```python
from build123d import *

# Parameters (mm, degrees)
F0_W     = 270
F0_H     = 270
F1_DEPTH = 240
F2_R     = 20
F3_T     = -2.5


with BuildPart() as f1:
    # F0 (on Top) → F1 (new body)
    with BuildSketch(Plane.XY):
        with Locations((137.330786, 0)):
            Rectangle(F0_W, F0_H)
    extrude(amount=-F1_DEPTH)

    # F2
    f2_edges = [f1.edges().sort_by_distance(p)[0] for p in [
        (137.330786, -135, -240),
        (272.330786, 0, -240),
        (137.330786, 135, -240),
        (2.330786, 0, -240),
        (2.330786, -135, -120),
        (272.330786, -135, -120),
        (272.330786, 135, -120),
        (2.330786, 135, -120),
    ]]
    fillet(f2_edges, radius=F2_R)

    # F3
    f3_openings = [f1.faces().sort_by_distance(p)[0] for p in [
        (137.330786, 0, 0),
    ]]
    offset(amount=F3_T, openings=f3_openings)


solid = f1.part
```
The listing builds one solid part. Answer for the finished solid, in the listing's coordinates (mm). A direction names the side the tool comes from. Coordinates: 2 decimals unless noted, no trailing zeros. Loops run counter-clockwise (first coordinate to the right, second up) from the corner with the lowest first, then second, coordinate; pieces in that order, holes last. Notation, with made-up numbers: (8.25, -27) -> (56.25, -27) arc R26 cw to (56.25, 5) -> close; hole circle Ø8 at (-19.75, 6.25). An arc over 180 degrees is marked (long way). Use one line per item in the form item = value. Start each with the question number.
Item 1: The part is cut by section A-A on z = -133. Determine the outline of the cut face in (x, y).
Item 2: Consider L1, parallel to Y at x = 216, z = -75.5; L2, parallel to X at y = 6, z = -121; L3, parallel to Z at x = 67, y = 112.5. Determine where each line is inside the solid, lowest interval first. Write a range as [from, to].
Item 3: The mould has two halves that part along Y. Classify faces 3 (the face through (266.628, 1.61, -233.986)), 4 (the face through (136, 135, -108)), 5 (the face through (264.84, 1.61, -232.24)): released by +Y, released by -Y, zero draft, split by the parting line, or undercut.
Item 4: The part is cut by section B-B on x = 49.5. Determine the outline of the cut face in (y, z), then the cut area to 3 significant figures.
Item 5: The part is cut by section C-C on y = -109. Determine the outline of the cut face in (x, z).
Item 6: A tool of negligible diameter and unlimited length cuts with its end or side. For faces 1 (the face through (269.831, -2, -108)), 2 (the face through (136, -135, -108)), from which of +Z, -Z, +X, -X, +Y, -Y can it reach the whole face along a straight path? Write none if from no direction.
Answer key:
q1.outline = (2.33, -115) arc R20 ccw to (22.33, -135) -> (252.33, -135) arc R20 ccw to (272.33, -115) -> (272.33, 115) arc R20 ccw to (252.33, 135) -> (22.33, 135) arc R20 ccw to (2.33, 115) -> close; hole (4.83, -115) arc R17.5 ccw to (22.33, -132.5) -> (252.33, -132.5) arc R17.5 ccw to (269.83, -115) -> (269.83, 115) arc R17.5 ccw to (252.33, 132.5) -> (22.33, 132.5) arc R17.5 ccw to (4.83, 115) -> close
q2.L1 = [-135, -132.5], [132.5, 135]
q2.L2 = [2.33, 4.83], [269.83, 272.33]
q2.L3 = [-240, -237.5]
q3.face_3 = zero draft
q3.face_4 = released by +Y
q3.face_5 = undercut
q4.outline = (-135, -220) arc R20 ccw to (-115, -240) -> (115, -240) arc R20 ccw to (135, -220) -> (135, 0) -> (132.5, 0) -> (132.5, -220) arc R17.5 cw to (115, -237.5) -> (-115, -237.5) arc R17.5 cw to (-132.5, -220) -> (-132.5, 0) -> (-135, 0) -> close
q4.area = 1,820 mm2
q5.outline = (2.33, -220) arc R20 ccw to (22.33, -240) -> (252.33, -240) arc R20 ccw to (272.33, -220) -> (272.33, 0) -> (269.83, 0) -> (269.83, -220) arc R17.5 cw to (252.33, -237.5) -> (22.33, -237.5) arc R17.5 cw to (4.83, -220) -> (4.83, 0) -> (2.33, 0) -> close
q6.face_1 = +Z
q6.face_2 = +Z, -Z, +X, -X, -Y
